from build123d import *

# Parameters (mm, degrees)
BOSS_EXTRUDE1_DEPTH = 90
CUT_EXTRUDE1_DEPTH  = 30


with BuildPart() as part:
    # Sketch1 → Boss-Extrude1 (new body)
    with BuildSketch(Plane(origin=(0, 0, 0), x_dir=(1, 0, 0), z_dir=(0, 1, 0))):
        with BuildLine():
            Line((6.409392014, -3), (6.409392014, 3))
            Line((6.409392014, 3), (9.539392014, 3))
            ThreePointArc((9.539392014, 3), (-10, 0), (9.539392014, -3))
            Line((9.539392014, -3), (6.409392014, -3))
        make_face()
        with BuildLine():
            Line((9.539392014, 3), (6.409392014, 3))
            Line((6.409392014, 3), (6.409392014, -3))
            Line((6.409392014, -3), (9.539392014, -3))
            ThreePointArc((9.539392014, -3), (9.884177258, -1.517576993), (10, 0))
            ThreePointArc((10, 0), (9.884177258, 1.517576993), (9.539392014, 3))
        make_face()
    extrude(amount=BOSS_EXTRUDE1_DEPTH)

    # Sketch1_3 → Cut-Extrude1 (cut)
    with BuildSketch(Plane(origin=(0, 0, 0), x_dir=(1, 0, 0), z_dir=(0, 1, 0))):
        with BuildLine():
            Line((9.539392014, 3), (6.409392014, 3))
            Line((6.409392014, 3), (6.409392014, -3))
            Line((6.409392014, -3), (9.539392014, -3))
            ThreePointArc((9.539392014, -3), (9.884177258, -1.517576993), (10, 0))
            ThreePointArc((10, 0), (9.884177258, 1.517576993), (9.539392014, 3))
        make_face()
    extrude(amount=CUT_EXTRUDE1_DEPTH, mode=Mode.SUBTRACT)


solid = part.part
Check sheet for the modelled part. Datum: model origin and axes. Units: mm. A direction names the side the tool comes from. Give positions to 0.01 mm unless a question says otherwise; leave off trailing zeros. Write each loop counter-clockwise with the first axis right and the second up, starting at its lowest first coordinate (ties: lowest second). Pieces come first, ordered by that corner, then holes. Notation, with made-up numbers: (69, 61) -> (99, 61) arc R23 cw to (99, 74) -> close; hole circle Ø11 at (48.5, 11.25). An arc over 180 degrees is marked (long way). One line per item, written item: value. Start each with the question number.
Item 1: Section check A-A on z = 8. Record the cut outline in (x, y), then the cut area to 3 significant figures.
Item 2: Gauge pin test, flat ends, axial feed: pin 1 (1.1 mm diameter, centred on x = 8, z = 1, fed in from -Y); pin 2 (3.5 mm diameter, centred on x = 8, y = 21, fed in from -Z); pin 3 (2 mm diameter, centred on y = 32.5, z = -2.5, fed in from -X). Record the tip position at first contact, or that the pin passes through.
Item 3: Tool access check on faces 1 (the flat face through (8, 15, 3)), 2 (the flat face through (0, 90, 0)). Record the directions out of +Z, -Z, +X, -X, +Y, -Y that give a thin tool (end or side, any length) a straight path to the whole face; none if there is none.
Item 4: Draft check along Z on faces 3 (the flat face through (0, 0, 0)), 4 (the flat face through (8, 30, 0)). Enter one of: +Z half, -Z half, draft (parallel to the pull), parting line (faces both ways), or undercut.
Item 5: Section check D-D on z = -1.75. Record the cut outline in (x, y), then the cut area to 3 significant figures.
Item 6: Section check C-C on y = 71. Record the cut outline in (x, z).
Item 7: Section check B-B on x = -6. Record the cut outline in (y, z).
Item 8: Material ranges on probe 1 along X at (y, z) = (56, -0.25); probe 2 along X at (y, z) = (51.5, 7); probe 3 along Z at (x, y) = (-2.75, 30), recorded low to high. Write a range as from..to.
Results list:
1. outline: (-6, 0) -> (6, 0) -> (6, 90) -> (-6, 90) -> close
1. area: 1,080 mm²
2. pin 1: y = 30
2. pin 2: z = -7.81
2. pin 3: x = -9.89
3. face 1: +X, -Y
3. face 2: +Z, -Z, +X, -X, +Y
4. face 3: draft
4. face 4: undercut
5. outline: (-9.85, 0) -> (6.41, 0) -> (6.41, 30) -> (9.85, 30) -> (9.85, 90) -> (-9.85, 90) -> close
5. area: 1,670 mm²
6. outline: circle Ø20 at (0, 0)
7. outline: (0, -8) -> (90, -8) -> (90, 8) -> (0, 8) -> close
8. probe 1: -10..10
8. probe 2: -7.14..7.14
8. probe 3: -9.61..9.61
